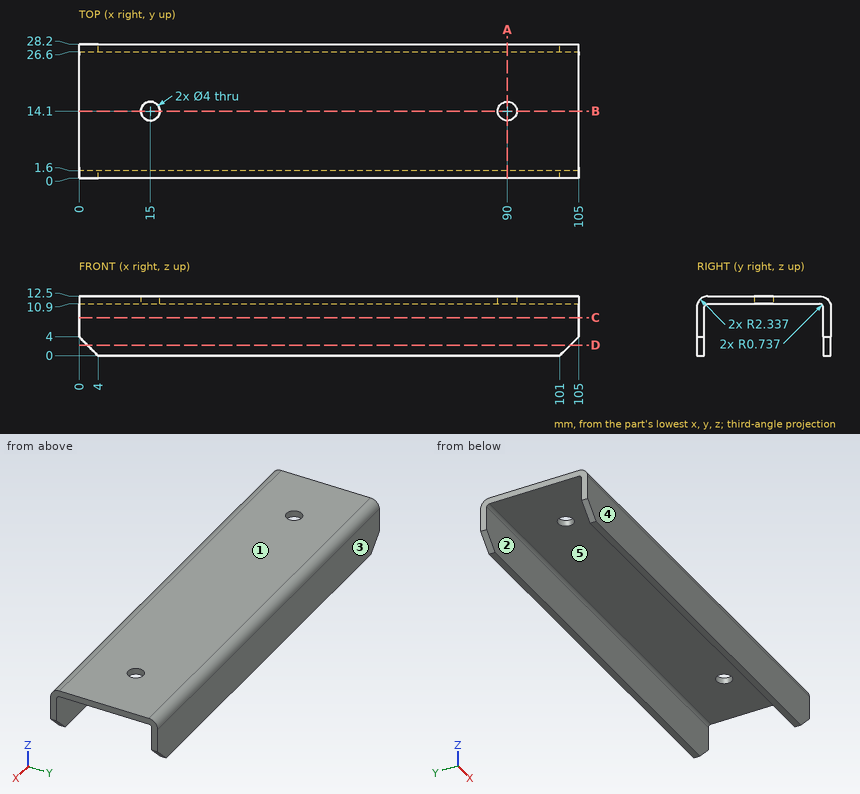
Input: dimensioned drawing with shaded views. Units: mm. Origin: part minimum x, y, z. A direction names the side the tool comes from. Coordinates: 2 decimals unless noted, no trailing zeros. Order: outer loops, then holes, each group sorted by start corner. A loop starts at its lowest first (then second) coordinate and runs counter-clockwise, first axis right, second up. Notation, with made-up numbers: (64, 86) - (73, 86) arc R17 ccw to (73, 99) - close; hole circle Ø7 at (-20, 61). An arc over 180 degrees is marked (long way). Put each result on its own line as item: value.
1. Line query: line 1 along Y through (x, z) = (88.5, 4.25); line 2 along Z through (x, y) = (51, 17); line 3 along Y through (x, z) = (15, 11.6) (1 decimal). Output: solid intervals per line, ascending.
Report:
line 1: y = 0 to 1.6, 26.6 to 28.2
line 2: z = 10.9 to 12.5
line 3: y = 0.5 to 12.1, 16.1 to 27.7
2. Cut plane A-A on x = 90. Return the cut outline in (y, z).
Report:
outline: (0, 0) - (1.6, 0) - (1.6, 10.16) arc R0.74 cw to (2.34, 10.9) - (12.1, 10.9) - (12.1, 12.5) - (2.34, 12.5) arc R2.34 ccw to (0, 10.16) - close; (16.1, 10.9) - (25.86, 10.9) arc R0.74 cw to (26.6, 10.16) - (26.6, 0) - (28.2, 0) - (28.2, 10.16) arc R2.34 ccw to (25.86, 12.5) - (16.1, 12.5) - close
3. Reachability of the marked faces 4 and 5 from +Z, -Z, +X, -X, +Y, -Y: full face, straight path, thin tool, end or side. Return the list, or none.
Report:
face 4: +Z, -Z, +X, -X, -Y
face 5: -Z, +X, -X
4. Contact query for flat-ended pins moving along their axis: pin 1 Ø3 at (x, y) = (15, 14.1) entering from +Z; pin 2 Ø12 at (x, y) = (70, 19.5) entering from -Z. Output: stop coordinate, or through.
Report:
pin 1: passes through
pin 2: stops at z = 10.9
5. Cut plane C-C on z = 8. Return the cut outline in (x, y).
Report:
outline: (0, 0) - (105, 0) - (105, 1.6) - (0, 1.6) - close; (0, 26.6) - (105, 26.6) - (105, 28.2) - (0, 28.2) - close
6. Cut plane B-B on y = 14.1. Return the cut outline in (x, z).
Report:
outline: (0, 10.9) - (13, 10.9) - (13, 12.5) - (0, 12.5) - close; (17, 10.9) - (88, 10.9) - (88, 12.5) - (17, 12.5) - close; (92, 10.9) - (105, 10.9) - (105, 12.5) - (92, 12.5) - close
7. Cut plane D-D on z = 2.25. Return the cut outline in (x, y).
Report:
outline: (1.75, 0) - (103.25, 0) - (103.25, 1.6) - (1.75, 1.6) - close; (1.75, 26.6) - (103.25, 26.6) - (103.25, 28.2) - (1.75, 28.2) - close
8. Draft query along Y for the marked faces 1, 2 and 3. Return one class per face: pulls with the +Y half, pulls with the -Y half, needs draft (parallel to the pull), parting line crosses it, or undercut.
Report:
face 1: needs draft
face 2: undercut
face 3: pulls with the +Y half
